Print and shaded views of the part. All mm, measured from the part's lowest x, y and z. Coordinates: 2 decimals unless noted, no trailing zeros. Loops run counter-clockwise (first coordinate to the right, second up) from the corner with the lowest first, then second, coordinate; pieces in that order, holes last.
1) Wall check: line 1 along X through (y, z) = (6, 81.5); line 2 along X through (y, z) = (1.75, 82.5) (1 decimal); line 3 along Z through (x, y) = (296, 1). Give the ranges that are in metal, low to high.
2) Saw through at A-A, the plane x = 40. Write the cut outline in (y, z) (1 decimal).
3) Saw through at B-B, the plane z = 92.5. Write the cut outline in (x, y), and give its area (3 significant figures).
4) Saw through at C-C, the plane y = 10.75. Write the cut outline in (x, z) (1 decimal), and give its area (3 significant figures).
5) Saw through at D-D, the plane x = 303. Write the cut outline in (y, z).
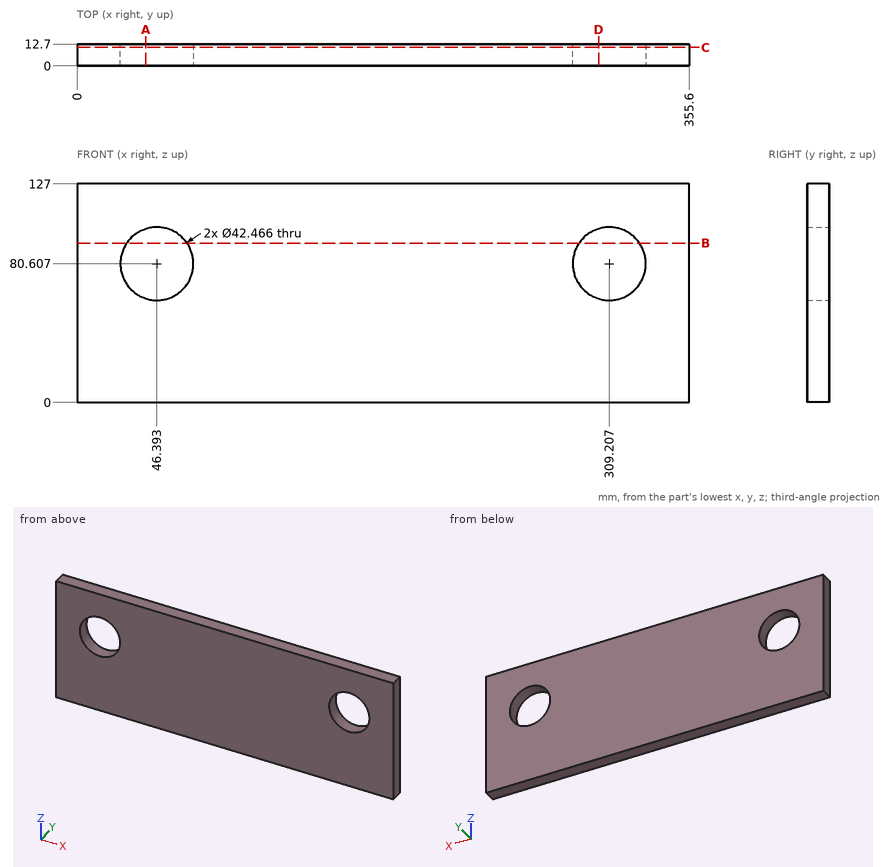
Data:
1. line 1: x = 0 to 25.18, 67.61 to 287.99, 330.42 to 355.6
1. line 2: x = 0 to 25.2, 67.5 to 288.1, 330.4 to 355.6
1. line 3: z = 0 to 63.98, 97.23 to 127
2. outline: (0, 0) - (12.7, 0) - (12.7, 60.4) - (0, 60.4) - close; (0, 100.9) - (12.7, 100.9) - (12.7, 127) - (0, 127) - close
3. outline: (0, 0) - (28.8, 0) - (28.8, 12.7) - (0, 12.7) - close; (63.98, 0) - (291.62, 0) - (291.62, 12.7) - (63.98, 12.7) - close; (326.8, 0) - (355.6, 0) - (355.6, 12.7) - (326.8, 12.7) - close
3. area: 3,620 mm2
4. outline: (0, 0) - (355.6, 0) - (355.6, 127) - (0, 127) - close; hole circle Ø42.5 at (46.4, 80.6); hole circle Ø42.5 at (309.2, 80.6)
4. area: 42,300 mm2
5. outline: (0, 0) - (12.7, 0) - (12.7, 60.3) - (0, 60.3) - close; (0, 100.91) - (12.7, 100.91) - (12.7, 127) - (0, 127) - close
